Verification items for the finished model (mm, model axes). Coordinates: 2 decimals unless noted, no trailing zeros. Answer as CSV lines item,"result". Start each with the question number.
1. Go/stop test with a flat-tipped pin: pin 1 (3 mm diameter, centred on x = 30, z = 55, fed in from +Y). Record where the tip stops, or that it passes through.
2. Material ranges on L1, parallel to X at y = 0.8, z = -55; L2, parallel to Z at x = -30, y = 0.9; L3, parallel to Z at x = -28.5, y = 1.8, recorded low to high. Write a range as [from, to].
3. Mould release check, pull along X, two halves, no side actions. Record for faces 1 (the cylindrical face through (28.16, 1.52, 56.69)), 2 (the flat face through (-2, 3, -1)), 3 (the cylindrical face through (-32.5, 1.5, -55.1)): pulls with the +X half, pulls with the -X half, needs draft (parallel to the pull), parting line crosses it, or undercut.
from build123d import *

# Parameters (mm, degrees)
SKETCH_1_W          = 300
SKETCH_1_H          = 140
EXTRUDE_1_DEPTH     = 3
SKETCH_2_R          = 2.5
CUT_EXTRUDE_1_DEPTH = 3


with BuildPart() as part:
    # 草图1 → 凸台-拉伸1 (new body)
    with BuildSketch(Plane(origin=(0, 0, 0), x_dir=(1, 0, 0), z_dir=(0, 1, 0))):
        Rectangle(SKETCH_1_W, SKETCH_1_H)
    extrude(amount=EXTRUDE_1_DEPTH)

    # 草图2 → 切除-拉伸1 (cut)
    with BuildSketch(Plane(origin=(0, 3, 0), x_dir=(1, 0, 0), z_dir=(0, 1, 0))):
        with Locations((-30, 55)):
            Circle(SKETCH_2_R)
        with Locations((30, 55)):
            Circle(SKETCH_2_R)
    cut_extrude_1 = extrude(amount=-CUT_EXTRUDE_1_DEPTH, mode=Mode.SUBTRACT)

    # 镜向1: 切除-拉伸1 across plane
    add(cut_extrude_1.mirror(Plane.XY), mode=Mode.SUBTRACT)


solid = part.part
Evaluation:
1,pin 1,"passes through"
2,L1,"x = [-150, -32.5], [-27.5, 27.5], [32.5, 150]"
2,L2,"z = [-70, -57.5], [-52.5, 52.5], [57.5, 70]"
2,L3,"z = [-70, -57], [-53, 53], [57, 70]"
3,face 1,"undercut"
3,face 2,"needs draft"
3,face 3,"undercut"
